from build123d import *

# Parameters (mm, degrees)
SKETCH2_R                                      = 330
SKETCH2_R_2                                    = 250
SKETCH2_W                                      = 44.45
SKETCH2_H                                      = 42
BOSS_EXTRUDE1_DEPTH                            = 12
CUT_EXTRUDE1_DEPTH                             = 12
SKETCH5_W                                      = 60
SKETCH5_H                                      = 60
CUT_EXTRUDE2_DEPTH                             = 12
FILLET1_R                                      = 5
SKETCH6_W                                      = 5
SKETCH6_H                                      = 30
CUT_EXTRUDE3_DEPTH                             = 12
FILLET2_R                                      = 3
CSK_FOR_M4_FLAT_HEAD_MACHINE_SCREW_D           = 4.5
CSK_FOR_M4_FLAT_HEAD_MACHINE_SCREW_CSINK_D     = 9.4
CSK_FOR_M4_FLAT_HEAD_MACHINE_SCREW_CSINK_ANGLE = 90


with BuildPart() as part:
    # Sketch2 → Boss-Extrude1 (new body)
    with BuildSketch(Plane.XY.offset(-518.360637908)):
        Circle(SKETCH2_R)
        Circle(SKETCH2_R_2, mode=Mode.SUBTRACT)
        with Locations((0, -303)):
            Rectangle(SKETCH2_W, SKETCH2_H, mode=Mode.SUBTRACT)
        Polygon((269.479730826, 181.247414599), (233.106663867, 160.247414599), (255.331663867, 121.752585401), (291.704730826, 142.752585401), align=None, mode=Mode.SUBTRACT)
        Polygon((-291.704730826, 142.752585401), (-255.331663867, 121.752585401), (-233.106663867, 160.247414599), (-269.479730826, 181.247414599), align=None, mode=Mode.SUBTRACT)
    extrude(amount=BOSS_EXTRUDE1_DEPTH)

    # Sketch3 → Cut-Extrude1 (cut)
    with BuildSketch(Plane.XY.offset(-506.360637908)):
        with BuildLine():
            Line((191.51111078, 160.696902422), (202.422805046, 169.852901056))
            ThreePointArc((202.422805046, 169.852901056), (209.542560602, 184.184300077), (203.874000238, 199.14917029))
            ThreePointArc((203.874000238, 199.14917029), (0, 285), (-203.874000238, 199.14917029))
            ThreePointArc((-203.874000238, 199.14917029), (-209.542560602, 184.184300077), (-202.422805046, 169.852901056))
            Line((-202.422805046, 169.852901056), (-191.51111078, 160.696902422))
            ThreePointArc((-191.51111078, 160.696902422), (0, 250), (191.51111078, 160.696902422))
        make_face()
        with BuildLine():
            Line((43.412044417, -246.201938253), (45.885524698, -260.229742003))
            ThreePointArc((45.885524698, -260.229742003), (54.737002544, -273.561330694), (70.531240495, -276.134648522))
            ThreePointArc((70.531240495, -276.134648522), (246.817240079, -142.5), (274.405240732, 76.985478232))
            ThreePointArc((274.405240732, 76.985478232), (264.279563146, 89.377030617), (248.308329744, 90.376840947))
            Line((248.308329744, 90.376840947), (234.923155196, 85.505035831))
            ThreePointArc((234.923155196, 85.505035831), (216.506350946, -125), (43.412044417, -246.201938253))
        make_face()
        with BuildLine():
            Line((-234.923155196, 85.505035831), (-248.308329744, 90.376840947))
            ThreePointArc((-248.308329744, 90.376840947), (-264.279563146, 89.377030617), (-274.405240732, 76.985478232))
            ThreePointArc((-274.405240732, 76.985478232), (-246.817240079, -142.5), (-70.531240495, -276.134648522))
            ThreePointArc((-70.531240495, -276.134648522), (-54.737002544, -273.561330694), (-45.885524698, -260.229742003))
            Line((-45.885524698, -260.229742003), (-43.412044417, -246.201938253))
            ThreePointArc((-43.412044417, -246.201938253), (-216.506350946, -125), (-234.923155196, 85.505035831))
        make_face()
    extrude(amount=-CUT_EXTRUDE1_DEPTH, mode=Mode.SUBTRACT)

    # Sketch5 → Cut-Extrude2 (cut)
    with BuildSketch(Plane.XY.offset(-506.360637908)):
        with Locations((0, 340)):
            Rectangle(SKETCH5_W, SKETCH5_H)
    extrude(amount=-CUT_EXTRUDE2_DEPTH, mode=Mode.SUBTRACT)

    # Fillet1
    fillet1_edges = [part.edges().sort_by_distance(p)[0] for p in [
        (30, 328.633534503, -512.360637908),
        (-30, 328.633534503, -512.360637908),
        (-30, 310, -512.360637908),
        (30, 310, -512.360637908),
    ]]
    fillet(fillet1_edges, radius=FILLET1_R)

    # Sketch6 → Cut-Extrude3 (cut)
    with BuildSketch(Plane.XY.offset(-506.360637908)):
        with Locations((0, 295)):
            Rectangle(SKETCH6_W, SKETCH6_H)
    extrude(amount=-CUT_EXTRUDE3_DEPTH, mode=Mode.SUBTRACT)

    # Fillet2
    fillet2_edges = [part.edges().sort_by_distance(p)[0] for p in [
        (2.5, 284.989034877, -512.360637908),
        (2.5, 310, -512.360637908),
        (-2.5, 284.989034877, -512.360637908),
        (-2.5, 310, -512.360637908),
    ]]
    fillet(fillet2_edges, radius=FILLET2_R)

    # CSK for M4 Flat Head Machine Screw (through all)
    with Locations(Plane(origin=(0, 0, -530.360637908), x_dir=(1, 0, 0), z_dir=(0, 0, -1))):
        with Locations((80.233903982, 299.43700615), (219.203102168, 219.203102168), (299.43700615, 80.233903982), (299.43700615, -80.233903982), (219.203102168, -219.203102168), (80.233903982, -299.43700615), (-80.233903982, -299.43700615), (-219.203102168, -219.203102168), (-299.43700615, -80.233903982), (-299.43700615, 80.233903982), (-219.203102168, 219.203102168), (-80.233903982, 299.43700615), (0, 0)):
            CounterSinkHole(CSK_FOR_M4_FLAT_HEAD_MACHINE_SCREW_D / 2, CSK_FOR_M4_FLAT_HEAD_MACHINE_SCREW_CSINK_D / 2, counter_sink_angle=CSK_FOR_M4_FLAT_HEAD_MACHINE_SCREW_CSINK_ANGLE)


solid = part.part
CAD build for the part. Positions are in the model's coordinates, mm. A direction names the side the tool comes from. Coordinates: 2 decimals unless noted, no trailing zeros. Order: outer loops, then holes, each group sorted by start corner. A loop starts at its lowest first (then second) coordinate and runs counter-clockwise, first axis right, second up. Notation, with made-up numbers: (33, -35.5) -> (86, -35.5) arc R25 cw to (86, -15.5) -> close; hole circle Ø2 at (-27, -2). An arc over 180 degrees is marked (long way). Answer in a Markdown table with one row per item.
1) Which spindle directions (+Z, -Z, +X, -X, +Y, -Y) get a long thin tool onto all of the face, cutting with end or side? Do faces 1 (the face through (-222, 122, -506.361)), 2 (the face through (-264.074, 89.481, -512.277)). Say none if no direction does.
Check values:
| item | result |
|---|---|
| face 1 | +Z, +X, -X, +Y, -Y |
| face 2 | +Z, -Z |
2) Mould opens along X. For faces 3 (the face through (-14.011, -329.702, -512.445)), 4 (the face through (273.264, 132.106, -512.445)), 5 (the face through (-222, 122, -518.361)) say: pulls with the +X half, pulls with the -X half, needs draft (parallel to the pull), parting line crosses it, or undercut.
Check values:
| item | result |
|---|---|
| face 3 | parting line crosses it |
| face 4 | undercut |
| face 5 | needs draft |
3) Band-saw the part on A-A (y = 0). List the corners of the cut face in (x, z).
Check values:
| item | result |
|---|---|
| outline | (-330, -518.36) -> (-285, -518.36) -> (-285, -506.36) -> (-330, -506.36) -> close; (285, -518.36) -> (330, -518.36) -> (330, -506.36) -> (285, -506.36) -> close |
4) Band-saw the part on C-C (y = 269). List the corners of the cut face in (x, z), and give its area (3 significant figures).
Check values:
| item | result |
|---|---|
| outline | (-191.15, -518.36) -> (-94.15, -518.36) -> (-94.15, -506.36) -> (-191.15, -506.36) -> close; (94.15, -518.36) -> (191.15, -518.36) -> (191.15, -506.36) -> (94.15, -506.36) -> close |
| area | 2,330 mm2 |
5) Flat gauge pins, fed straight in: P1, Ø3, axis at y = -195, z = -516.5, coming from the +X side; P2, Ø2, axis at x = -176.5, z = -509, coming from the -Y side; P3, Ø2.5, axis at x = 80.23, y = 299.44, coming from the -Z side; P4, Ø3, axis at y = -170, z = -508.5, coming from the -X side. Where does each tip first touch, or does it go through?
Check values:
| item | result |
|---|---|
| P1 | x = 267.32 |
| P2 | y = -279.46 |
| P3 | through |
| P4 | x = -283.74 |
6) Drill centre lines: line 1 (Y direction, x = -15.5, z = -511.5); line 2 (Y direction, x = 246.5, z = -512.25); line 3 (X direction, y = -50.5, z = -515.25). Where is each one in solid material? Low to high.
Check values:
| item | result |
|---|---|
| line 1 | -329.64 to -324, -282 to -249.52, 284.58 to 310 |
| line 2 | -219.4 to -143.05, 89.72 to 137.05, 167.98 to 219.4 |
| line 3 | -326.11 to -280.49, 280.49 to 326.11 |
7) Band-saw the part on B-B (z = -513.5). Give the number of separate pieces and of enclosed holes in the cut face, and give its area (3 significant figures).
Check values:
| item | result |
|---|---|
| separate pieces | 1 |
| enclosed holes | 15 |
| area | 90,200 mm2 |
